Source: CAD feature listing. Evaluate the final solid. Frame: model axes, mm. Round coordinates to 2 decimals unless told otherwise and drop trailing zeros. Loops run counter-clockwise (first coordinate to the right, second up) from the corner with the lowest first, then second, coordinate; pieces in that order, holes last. Notation, with made-up numbers: (27.5, 59.5) -> (38.5, 59.5) arc R15 ccw to (38.5, 78.5) -> close; hole circle Ø10 at (44, -17.5). An arc over 180 degrees is marked (long way). Put each result on its own line as item: value. Start each with the question number.
1. Cut plane C-C (x = -53.5). Return the cut outline in (y, z), then the cut area to 3 significant figures.
2. Cut plane A-A (x = 40). Return the cut outline in (y, z).
3. Material intervals for L1, parallel to Y at x = -76, z = 3.85; L2, parallel to X at y = 5.75, z = 1.15; L3, parallel to X at y = -8.25, z = 0.7, sorted ascending.
4. Cut plane B-B (x = -2). Return the cut outline in (y, z), then the cut area to 3 significant figures.
5. Contact query for flat-ended pins moving along their axis: pin 1 (3 mm diameter, centred on x = -35.5, z = 2, fed in from -Y); pin 2 (1 mm diameter, centred on x = -23, z = 3, fed in from +Y). Output: stop coordinate, or through.
```python
from build123d import *

# Parameters (mm, degrees)
BOX003_W     = 40
BOX003_H     = 2
BOX003_DEPTH = 10
BOX004_W     = 40
BOX004_H     = 2
BOX004_DEPTH = 10
BOX002_W     = 40
BOX002_H     = 2
BOX002_DEPTH = 10
BOX005_W     = 50
BOX005_H     = 6
BOX005_DEPTH = 10
BOX006_W     = 50
BOX006_H     = 6
BOX006_DEPTH = 10
BOX001_W     = 40
BOX001_H     = 2
BOX001_DEPTH = 10
BOX_W        = 180
BOX_H        = 28
BOX_DEPTH    = 6
FILLET_R     = 5.99
FILLET001_R  = 2


with BuildPart() as cube003:
    # Box003 → Box003 (new body)
    with BuildSketch(Plane(origin=(20, -6, 0), x_dir=(1, 0, 0), z_dir=(0, 0, 1))):
        with Locations((20, 1)):
            Rectangle(BOX003_W, BOX003_H)
    extrude(amount=BOX003_DEPTH)


with BuildPart() as cube004:
    # Box004 → Box004 (new body)
    with BuildSketch(Plane(origin=(20, 4, 0), x_dir=(1, 0, 0), z_dir=(0, 0, 1))):
        with Locations((20, 1)):
            Rectangle(BOX004_W, BOX004_H)
    extrude(amount=BOX004_DEPTH)


with BuildPart() as cube002:
    # Box002 → Box002 (new body)
    with BuildSketch(Plane(origin=(-100, 4, 0), x_dir=(1, 0, 0), z_dir=(0, 0, 1))):
        with Locations((20, 1)):
            Rectangle(BOX002_W, BOX002_H)
    extrude(amount=BOX002_DEPTH)


with BuildPart() as cube005:
    # Box005 → Box005 (new body)
    with BuildSketch(Plane(origin=(-45, -14, 0), x_dir=(1, 0, 0), z_dir=(0, 0, 1))):
        with Locations((25, 3)):
            Rectangle(BOX005_W, BOX005_H)
    extrude(amount=BOX005_DEPTH)


with BuildPart() as cube006:
    # Box006 → Box006 (new body)
    with BuildSketch(Plane(origin=(-45, 8, 0), x_dir=(1, 0, 0), z_dir=(0, 0, 1))):
        with Locations((25, 3)):
            Rectangle(BOX006_W, BOX006_H)
    extrude(amount=BOX006_DEPTH)


with BuildPart() as holes:
    # Box001 → Box001 (new body)
    with BuildSketch(Plane(origin=(-100, -6, 0), x_dir=(1, 0, 0), z_dir=(0, 0, 1))):
        with Locations((20, 1)):
            Rectangle(BOX001_W, BOX001_H)
    extrude(amount=BOX001_DEPTH)

    # Fusion: union Cube003, Cube004, Cube002, Cube005, Cube006
    add(cube003.part)
    add(cube004.part)
    add(cube002.part)
    add(cube005.part)
    add(cube006.part)


with BuildPart() as fillet001:
    # Box → Box (new body)
    with BuildSketch(Plane(origin=(-110, -14, 0), x_dir=(1, 0, 0), z_dir=(0, 0, 1))):
        with Locations((90, 14)):
            Rectangle(BOX_W, BOX_H)
    extrude(amount=BOX_DEPTH)

    # Cut: cut Holes
    add(holes.part, mode=Mode.SUBTRACT)

    # Fillet
    fillet_edges = [fillet001.edges().sort_by_distance(p)[0] for p in [
        (-110, -14, 3),
        (-110, 14, 3),
        (-45, -14, 3),
        (-45, 14, 3),
        (5, 14, 3),
        (70, 14, 3),
        (70, -14, 3),
        (5, -14, 3),
    ]]
    fillet(fillet_edges, radius=FILLET_R)

    # Fillet001
    fillet001_edges = [fillet001.edges().sort_by_distance(p)[0] for p in [
        (-110, 0, 6),
        (-110, 0, 0),
        (-77.5, 14, 6),
        (-108.24557, 12.24557, 6),
        (-46.75443, 12.24557, 6),
        (-108.24557, -12.24557, 6),
        (-20, 8, 6),
        (-77.5, -14, 6),
        (-46.75443, -12.24557, 6),
        (6.75443, 12.24557, 6),
        (37.5, 14, 6),
        (-20, -8, 6),
        (68.24557, 12.24557, 6),
        (70, 0, 6),
        (6.75443, -12.24557, 6),
        (68.24557, -12.24557, 6),
        (37.5, -14, 6),
        (-80, -6, 6),
        (-80, -4, 6),
        (-80, 4, 6),
        (-80, 6, 6),
        (40, 4, 6),
        (40, 6, 6),
        (40, -6, 6),
        (40, -4, 6),
        (-108.24557, -12.24557, 0),
        (-108.24557, 12.24557, 0),
        (-77.5, 14, 0),
        (-46.75443, 12.24557, 0),
        (-20, 8, 0),
        (-77.5, -14, 0),
        (-46.75443, -12.24557, 0),
        (6.75443, 12.24557, 0),
        (37.5, 14, 0),
        (-20, -8, 0),
        (68.24557, 12.24557, 0),
        (70, 0, 0),
        (6.75443, -12.24557, 0),
        (68.24557, -12.24557, 0),
        (37.5, -14, 0),
        (-80, -6, 0),
        (-80, -4, 0),
        (-80, 4, 0),
        (-80, 6, 0),
        (40, 4, 0),
        (40, 6, 0),
        (40, -6, 0),
        (40, -4, 0),
    ]]
    fillet(fillet001_edges, radius=FILLET001_R)


solid = fillet001.part
```
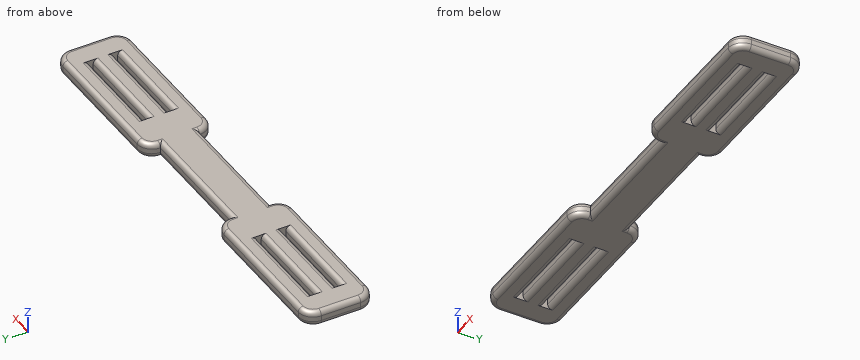
Solution:
1. outline: (-14, 2) arc R2 ccw to (-12, 0) -> (12, 0) arc R2 ccw to (14, 2) -> (14, 4) arc R2 ccw to (12, 6) -> (-12, 6) arc R2 ccw to (-14, 4) -> close
1. area: 165 mm^2
2. outline: (-14, 2) arc R2 ccw to (-12, 0) -> (-8, 0) arc R2 ccw to (-6, 2) -> (-6, 4) arc R2 ccw to (-8, 6) -> (-12, 6) arc R2 ccw to (-14, 4) -> close; (-4, 2) arc R2 ccw to (-2, 0) -> (2, 0) arc R2 ccw to (4, 2) -> (4, 4) arc R2 ccw to (2, 6) -> (-2, 6) arc R2 ccw to (-4, 4) -> close; (6, 2) arc R2 ccw to (8, 0) -> (12, 0) arc R2 ccw to (14, 2) -> (14, 4) arc R2 ccw to (12, 6) -> (8, 6) arc R2 ccw to (6, 4) -> close
3. L1: y = -14 to -6, -4 to 4, 6 to 14
3. L2: x = -109.81 to -100, -60 to 20, 60 to 69.81
3. L3: x = -109.51 to -45.49, 5.49 to 69.51
4. outline: (-8, 2) arc R2 ccw to (-6, 0) -> (6, 0) arc R2 ccw to (8, 2) -> (8, 4) arc R2 ccw to (6, 6) -> (-6, 6) arc R2 ccw to (-8, 4) -> close
4. area: 92.6 mm^2
5. pin 1: stops at y = -8
5. pin 2: stops at y = 8
